Geometry: final body of the model. Coordinates: model frame, mm. A direction names the side the tool comes from. Give positions to 0.01 mm unless a question says otherwise; leave off trailing zeros. Loops run counter-clockwise (first coordinate to the right, second up) from the corner with the lowest first, then second, coordinate; pieces in that order, holes last.
```python
from build123d import *

# Parameters (mm, degrees)
BOSS_EXTRUDE2_DEPTH = 15
FILLET1_R           = 3.33
SKETCH3_W           = 80
SKETCH3_H           = 22.592249713
BOSS_EXTRUDE3_DEPTH = 110
SKETCH4_W           = 80
SKETCH4_H           = 25.180318724
SKETCH4_H_2         = 19.389592809
SKETCH4_H_3         = 23.819220414
BOSS_EXTRUDE4_DEPTH = 110
FILLET2_R           = 7.5
SKETCH5_RX          = 31.460220339
SKETCH5_RY          = 15.185408179
CUT_EXTRUDE1_DEPTH  = 10


with BuildPart() as part:
    # Sketch2 → Boss-Extrude2 (new, symmetric)
    with BuildSketch(Plane.XY):
        Polygon((80, 244), (80, 56.32), (80, 0), (0, 0), (0, 244), align=None)
        Polygon((149.68, 56.32), (80, 56.32), (80, 19.389592809), (149.68, 19.389592809), (149.68, 25.879592809), (110.31, 25.879592809), (110.31, 49.83), (149.68, 49.83), align=None)
    extrude(amount=BOSS_EXTRUDE2_DEPTH, both=True)

    # Fillet1
    # the kernel refuses this fillet: 3.33 mm, written as the material it takes off along each edge
    with BuildSketch(Plane(origin=(149.68, 19.389592809, -23.325), x_dir=(-1, 0, 0), z_dir=(0, 0, 1)), Plane(origin=(149.68, 25.879592809, -23.325), x_dir=(0, -1, 0), z_dir=(0, 0, 1)), Plane(origin=(149.68, 49.83, 23.325), x_dir=(0, 1, 0), z_dir=(0, 0, -1)), Plane(origin=(149.68, 56.32, 23.325), x_dir=(-1, 0, 0), z_dir=(0, 0, -1))) as fillet1_piece_1:
        with BuildLine():
            CenterArc((FILLET1_R, -FILLET1_R), FILLET1_R, 90, 90)
            Line((0, -FILLET1_R), (0, 0))
            Line((0, 0), (FILLET1_R, 0))
        make_face()
    extrude(amount=46.65, mode=Mode.SUBTRACT)

    # Sketch3 → Boss-Extrude3 (add)
    with BuildSketch(Plane.XY):
        with Locations((40, 232.703875144)):
            Rectangle(SKETCH3_W, SKETCH3_H)
    extrude(amount=BOSS_EXTRUDE3_DEPTH)

    # Sketch4 → Boss-Extrude4 (add)
    with BuildSketch(Plane.XY):
        with Locations((40, 179.676540861)):
            Rectangle(SKETCH4_W, SKETCH4_H)
        with Locations((40, 9.694796404)):
            Rectangle(SKETCH4_W, SKETCH4_H_2)
        with Locations((40, 42.545886188)):
            Rectangle(SKETCH4_W, SKETCH4_H_3)
    extrude(amount=BOSS_EXTRUDE4_DEPTH)

    # Fillet2
    fillet2_edges = [part.edges().sort_by_distance(p)[0] for p in [
        (40, 167.086381499, 110),
        (40, 192.266700223, 110),
        (40, 0, 110),
        (40, 19.389592809, 110),
        (40, 30.636275981, 110),
        (40, 54.455496395, 110),
        (40, 221.407750287, 110),
        (40, 244, 110),
    ]]
    fillet(fillet2_edges, radius=FILLET2_R)

    # Sketch5 → Cut-Extrude1 (cut)
    with BuildSketch(Plane.XY.offset(15)):
        with Locations(Location((37.068979408, 133.739472919), (0, 0, -38.85337434))):
            Ellipse(SKETCH5_RX, SKETCH5_RY)
    extrude(amount=-CUT_EXTRUDE1_DEPTH, mode=Mode.SUBTRACT)


solid = part.part
```
Q1. Section query A-A, the plane x = 135. Return loops of the section in (y, z), and give its area (3 significant figures).
Q2. Section query D-D, the plane x = 86. Return loops of the section in (y, z).
Q3. Section query B-B, the plane z = 89. Return loops of the section in (x, y).
Q4. Pin query (flat end, axial travel): pin 1 Ø14 at (x, y) = (34, 125) entering from +Z; pin 2 Ø15 at (x, z) = (122.5, 4.5) entering from +Y; pin 3 Ø9.5 at (y, z) = (10.5, 21) entering from +X. Return the tip coordinate at first contact, or that it passes through.
Q5. Mould query, pull axis Y, two halves, no side actions, for faces 5 (the face through (39, 43, 110)), 6 (the face through (39, 192.267, 58)), 7 (the face through (39, 244, 45)). Classes: +Y half, -Y half, draft (parallel to the pull), parting line (faces both ways), or undercut.
Q6. Section query C-C, the plane y = 218. Return loops of the section in (x, z), and give its area (3 significant figures).
Q7. Reachability of faces 1 (the face through (80, 170, 34)), 2 (the face through (80, 42, 62)), 3 (the face through (41, 207, 15)), 4 (the face through (110.31, 38, 0)) from +Z, -Z, +X, -X, +Y, -Y: full face, straight path, thin tool, end or side. Return the list, or none.
Q8. Material intervals for probe 1 along Y at (x, z) = (49.5, 87); probe 2 along Y at (x, z) = (139, 8); probe 3 along Z at (x, y) = (14.5, 29.5), sorted ascending.
Resolved:
1. outline: (19.39, -15) - (25.88, -15) - (25.88, 15) - (19.39, 15) - close; (49.83, -15) - (56.32, -15) - (56.32, 15) - (49.83, 15) - close
1. area: 389 mm2
2. outline: (19.39, -15) - (56.32, -15) - (56.32, 15) - (19.39, 15) - close
3. outline: (0, 0) - (80, 0) - (80, 19.39) - (0, 19.39) - close; (0, 30.64) - (80, 30.64) - (80, 54.46) - (0, 54.46) - close; (0, 167.09) - (80, 167.09) - (80, 192.27) - (0, 192.27) - close; (0, 221.41) - (80, 221.41) - (80, 244) - (0, 244) - close
4. pin 1: stops at z = 15
4. pin 2: stops at y = 56.32
4. pin 3: stops at x = 80
5. face 5: draft
5. face 6: undercut
5. face 7: +Y half
6. outline: (0, -15) - (80, -15) - (80, 15) - (0, 15) - close
6. area: 2,400 mm2
7. face 1: +Z, -Z, +X, +Y
7. face 2: +Z, +X, +Y, -Y
7. face 3: +Z, +X, -X
7. face 4: +Z, -Z, +X
8. probe 1: y = 0 to 19.39, 30.64 to 54.46, 167.09 to 192.27, 221.41 to 244
8. probe 2: y = 19.39 to 25.88, 49.83 to 56.32
8. probe 3: z = -15 to 15
